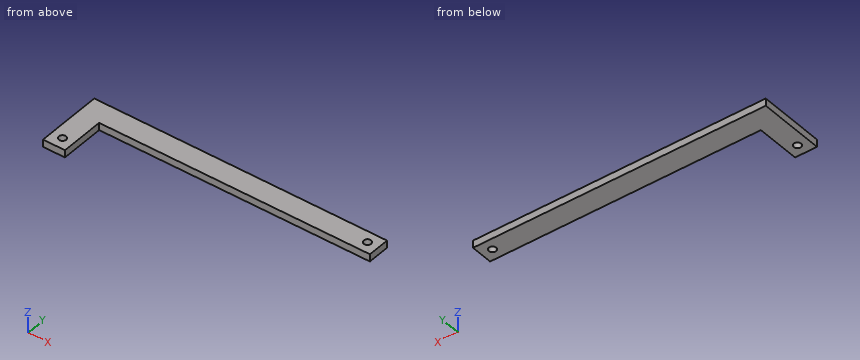
from build123d import *

# Parameters (mm, degrees)
SKETCH1_W           = 254
SKETCH1_H           = 19.05
SKETCH1_R           = 3.175
SKETCH1_W_2         = 19.05
SKETCH1_H_2         = 38.1
BOSS_EXTRUDE1_DEPTH = 6.35


with BuildPart() as part:
    # Sketch1 → Boss-Extrude1 (new body)
    # profile 1 of 2: a face of its own
    with BuildSketch(Plane.XY):
        with Locations((127, 9.525)):
            Rectangle(SKETCH1_W, SKETCH1_H)
        with Locations((244.475, 9.525)):
            Circle(SKETCH1_R, mode=Mode.SUBTRACT)
    # profile 2 of 2: a face of its own
    with BuildSketch(Plane.XY):
        with Locations((9.525, -19.05)):
            Rectangle(SKETCH1_W_2, SKETCH1_H_2)
        with Locations((9.525, -28.575)):
            Circle(SKETCH1_R, mode=Mode.SUBTRACT)
    extrude(amount=BOSS_EXTRUDE1_DEPTH)


solid = part.part
Work out the finished part from the listing and answer in its coordinate system (mm). Give positions to 0.01 mm unless a question says otherwise; leave off trailing zeros. Order: outer loops, then holes, each group sorted by start corner. A loop starts at its lowest first (then second) coordinate and runs counter-clockwise, first axis right, second up. Notation, with made-up numbers: (6, 75.5) -> (57, 75.5) arc R15 cw to (57, 93.5) -> close; hole circle Ø9 at (-27.5, -14.5). An arc over 180 degrees is marked (long way). One line per item, written item: value.
Item 1: Flat-ended cylindrical pins translate along their axes: P1, Ø4, axis at x = 244.475, y = 9.525, coming from the -Z side; P2, Ø3, axis at y = -17, z = 3.5, coming from the +X side. Find the tip coordinate at first contact, or state that the pin passes through.
Answer sheet:
P1: through
P2: x = 19.05
Item 2: Straight lines are drawn through the part: probe 1 along X at (y, z) = (-15, 4); probe 2 along X at (y, z) = (-27.5, 3). For each, find the intervals that lie inside material, in ascending order.
Answer sheet:
probe 1: 0 to 19.05
probe 2: 0 to 6.54, 12.51 to 19.05
Item 3: Find section A-A, the plane z = 3. Give the vertices of the cut face in (x, y) (3 decimals), plus the area to 3 significant figures.
Answer sheet:
outline: (0, -38.1) -> (19.05, -38.1) -> (19.05, 0) -> (254, 0) -> (254, 19.05) -> (0, 19.05) -> close; hole circle Ø6.35 at (9.525, -28.575); hole circle Ø6.35 at (244.475, 9.525)
area: 5,500 mm²
Item 4: Find section B-B, the plane y = -7.5. Give the vertices of the cut face in (x, z), plus the area to 3 significant figures.
Answer sheet:
outline: (0, 0) -> (19.05, 0) -> (19.05, 6.35) -> (0, 6.35) -> close
area: 121 mm²
